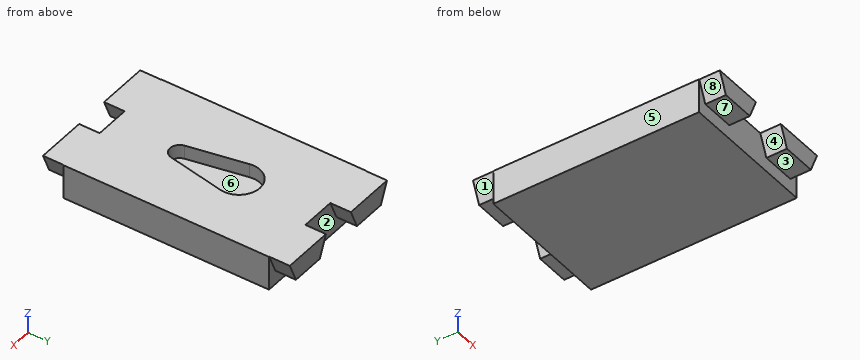
```python
from build123d import *

# Parameters (mm, degrees)
SKETCH_W     = 40
SKETCH_H     = 60
PAD_DEPTH    = 10
PAD001_DEPTH = 6
PAD002_DEPTH = 6
POCKET_DEPTH = 4


with BuildPart() as part:
    # Sketch → Pad (new body)
    with BuildSketch(Plane.XY):
        with Locations((20, 30)):
            Rectangle(SKETCH_W, SKETCH_H)
    extrude(amount=PAD_DEPTH)

    # Sketch001 (on Face3 of Pad) → Pad001 (join)
    with BuildSketch(Plane.XZ):
        Polygon((0.1, 10), (14.9, 10), (12.4, 4.1), (2.6, 4.1), align=None)
        Polygon((25.1, 10), (39.9, 10), (37.4, 4.1), (27.6, 4.1), align=None)
    extrude(amount=PAD001_DEPTH)

    # Sketch002 (on Face1 of Pad001) → Pad002 (join)
    with BuildSketch(Plane(origin=(0, 60, 0), x_dir=(-1, 0, 0), z_dir=(0, 1, 0))):
        Polygon((-39.9, 10), (-25.1, 10), (-27.6, 4.1), (-37.4, 4.1), align=None)
        Polygon((-14.9, 10), (-0.1, 10), (-2.6, 4.1), (-12.4, 4.1), align=None)
    extrude(amount=PAD002_DEPTH)

    # Sketch003 (on Face4 of Pad002) → Pocket (cut)
    with BuildSketch(Plane.XY.offset(10)):
        with BuildLine():
            ThreePointArc((25.987994, 35.836416), (20, 43.1), (14.012006, 35.836416))
            Line((14.012006, 35.836416), (17.251413, 19.165896))
            ThreePointArc((17.251413, 19.165896), (20, 16.9), (22.748587, 19.165896))
            Line((25.987994, 35.836416), (22.748587, 19.165896))
        make_face()
    extrude(amount=-POCKET_DEPTH, mode=Mode.SUBTRACT)


solid = part.part
```
Geometry check sheet. Reference: the model listing, model coordinates, mm. Face numbers are marked on the shaded views. A direction names the side the tool comes from. Coordinates: 2 decimals unless noted, no trailing zeros. Order: outer loops, then holes, each group sorted by start corner. A loop starts at its lowest first (then second) coordinate and runs counter-clockwise, first axis right, second up.
Item 1: Scan lines: line 1 along Y through (x, z) = (20, 8.35); line 2 along X through (y, z) = (37, 8.5); line 3 along Y through (x, z) = (8, 1). Record each from-to range of solid material in increasing order.
Item 2: Section check A-A (x = 9). Enter the section's corners in (y, z).
Item 3: Section check D-D (z = 1). Enter the section's corners in (x, y).
Item 4: Section check B-B (z = 8.75). Enter the section's corners in (x, y), plus the area to 3 significant figures.
Item 5: Mould release check, pull along X, two halves, no side actions. Record for the marked faces 1, 2 and 3: released by +X, released by -X, zero draft, split by the parting line, or undercut.
Item 6: Section check C-C (y = 37). Enter the section's corners in (x, z).
Item 7: Depth check by flat-ended pin: pin 1 (10 mm diameter, centred on x = 20, y = 37, fed in from +Z); pin 2 (1 mm diameter, centred on x = 15.5, z = 3, fed in from -Y); pin 3 (3 mm diameter, centred on x = 34, y = -2.5, fed in from -Z). Enter the tip coordinate at first touch or a pass-through.
Item 8: Tool access check on the marked faces 4, 5, 6, 7 and 8. Record the directions out of +Z, -Z, +X, -X, +Y, -Y that give a thin tool (end or side, any length) a straight path to the whole face; none if there is none.
Check sheet entries:
1. line 1: y = 0 to 16.9, 43.1 to 60
1. line 2: x = 0 to 13.9, 26.1 to 40
1. line 3: y = 0 to 60
2. outline: (-6, 4.1) - (0, 4.1) - (0, 0) - (60, 0) - (60, 4.1) - (66, 4.1) - (66, 10) - (-6, 10) - close
3. outline: (0, 0) - (40, 0) - (40, 60) - (0, 60) - close
4. outline: (0, 0) - (0.63, 0) - (0.63, -6) - (14.37, -6) - (14.37, 0) - (25.63, 0) - (25.63, -6) - (39.37, -6) - (39.37, 0) - (40, 0) - (40, 60) - (39.37, 60) - (39.37, 66) - (25.63, 66) - (25.63, 60) - (14.37, 60) - (14.37, 66) - (0.63, 66) - (0.63, 60) - (0, 60) - close; hole (14.01, 35.84) - (17.25, 19.17) arc R2.8 ccw to (22.75, 19.17) - (25.99, 35.84) arc R6.1 ccw (long way) to start
4. area: 2,500 mm2
5. face 1: released by -X
5. face 2: undercut
5. face 3: zero draft
6. outline: (0, 0) - (40, 0) - (40, 10) - (26.1, 10) - (26.1, 6) - (13.9, 6) - (13.9, 10) - (0, 10) - close
7. pin 1: stops at z = 6
7. pin 2: stops at y = 0
7. pin 3: stops at z = 4.1
8. face 4: -Z, -Y
8. face 5: +Z, -Z, -X, +Y, -Y
8. face 6: +Z
8. face 7: -Z, +X, -X, -Y
8. face 8: -Z, -X, -Y
